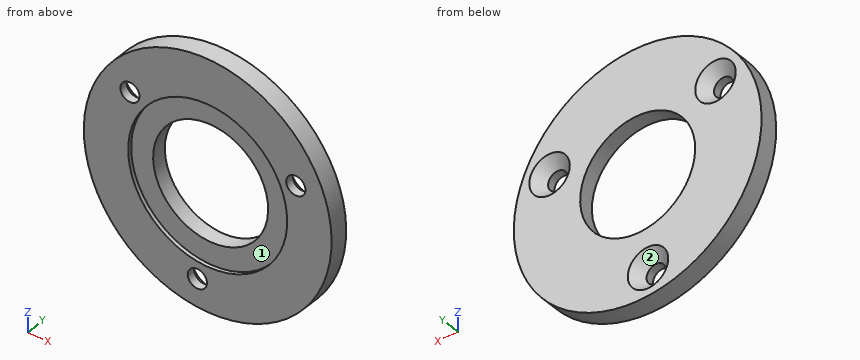
```python
from build123d import *

# Parameters (mm, degrees)
CSK_FOR_M3_SFHCS1_AT_2_COUNT = 2
CSK_FOR_M3_SFHCS1_AT_2_PITCH = 16.002
CSK_FOR_M3_SFHCS1_AT_3_COUNT = 2
CSK_FOR_M3_SFHCS1_AT_3_PITCH = 16.002
CSK_FOR_M3_SFHCS1_AT_4_COUNT = 2
CSK_FOR_M3_SFHCS1_AT_4_PITCH = 16.002


with BuildPart() as part:
    # Sketch1 → Revolve1 (revolve)
    with BuildSketch(Plane.XY, mode=Mode.PRIVATE) as revolve1_sk:
        Polygon((-9.5504, 0), (-20.574, 0), (-20.574, -3.1496), (-13.208, -3.1496), (-13.208, -2.5146), (-9.5504, -2.5146), align=None)
    revolve(revolve1_sk.sketch.rotate(Axis((0, 0, 0), (0, 1, 0)), 270), axis=Axis((0, 0, 0), (0, 1, 0)))

    # Sketch2 → CSK for M3 SFHCS1 (revolve, cut)
    with BuildSketch(Plane(origin=(0, 0, 0), x_dir=(0, 0, 1), z_dir=(1, 0, 0))):
        Polygon((0, 0), (0, 3.1496), (1.6, 3.1496), (1.6, 1.76), (3.36, 0), align=None)
    csk_for_m3_sfhcs1 = revolve(axis=Axis((0, 6.35, 0), (0, -1, 0)), mode=Mode.SUBTRACT)

    # CSK for M3 SFHCS1 at 2: CSK for M3 SFHCS1 ×2
    with Locations(*[Vector(-0.10721238743656843, 0, -0.9942361409545275) * (i * CSK_FOR_M3_SFHCS1_AT_2_PITCH) for i in range(1, CSK_FOR_M3_SFHCS1_AT_2_COUNT)]):
        add(csk_for_m3_sfhcs1, mode=Mode.SUBTRACT)

    # CSK for M3 SFHCS1 at 3: CSK for M3 SFHCS1 ×2
    with Locations(*[Vector(0.9146399491455367, 0, 0.4042694193567579) * (i * CSK_FOR_M3_SFHCS1_AT_3_PITCH) for i in range(1, CSK_FOR_M3_SFHCS1_AT_3_COUNT)]):
        add(csk_for_m3_sfhcs1, mode=Mode.SUBTRACT)

    # CSK for M3 SFHCS1 at 4: CSK for M3 SFHCS1 ×2
    with Locations(*[Vector(-0.8074275617089052, 0, 0.5899667215977628) * (i * CSK_FOR_M3_SFHCS1_AT_4_PITCH) for i in range(1, CSK_FOR_M3_SFHCS1_AT_4_COUNT)]):
        add(csk_for_m3_sfhcs1, mode=Mode.SUBTRACT)


solid = part.part
```
Build history of the part. All positions in model axes, mm. Face numbers are marked on the shaded views. A direction names the side the tool comes from. Round coordinates to 2 decimals unless told otherwise and drop trailing zeros. Order: outer loops, then holes, each group sorted by start corner. A loop starts at its lowest first (then second) coordinate and runs counter-clockwise, first axis right, second up. Notation, with made-up numbers: (28, 0.5) -> (74, 0.5) arc R21 cw to (74, 17.5) -> close; hole circle Ø10 at (-28, 39). An arc over 180 degrees is marked (long way). Answer in a Markdown table with one row per item.
1) Band-saw the part on D-D on z = -11.5. Give the cut face in (x, y), and give its area (3 significant figures).
Values:
| item | result |
|---|---|
| outline | (-17.06, -3.15) -> (-6.5, -3.15) -> (-6.5, -2.51) -> (6.5, -2.51) -> (6.5, -3.15) -> (17.06, -3.15) -> (17.06, 0) -> (-17.06, 0) -> close |
| area | 99.2 mm2 |
2) Band-saw the part on C-C on y = -0.7. Give the cut face in (x, z).
Values:
| item | result |
|---|---|
| outline | circle Ø41.15 at (0, 0); hole circle Ø5.32 at (-12.92, 9.44); hole circle Ø19.1 at (0, 0); hole circle Ø5.32 at (-1.72, -15.91); hole circle Ø5.32 at (14.64, 6.47) |
3) Band-saw the part on B-B on x = 8.5. Give the cut face in (y, z).
Values:
| item | result |
|---|---|
| outline | (-3.15, -18.74) -> (0, -18.74) -> (0, -4.35) -> (-2.51, -4.35) -> (-2.51, -10.11) -> (-3.15, -10.11) -> close; (-3.15, 10.11) -> (-2.51, 10.11) -> (-2.51, 4.35) -> (0, 4.35) -> (0, 18.74) -> (-3.15, 18.74) -> close |
4) Pin check, flat tips, straight feed: P1, Ø2.5, axis at x = -1.72, z = -15.91, coming from the -Y side; P2, Ø1.5, axis at y = -1, z = -6, coming from the +X side. Stop position of each tip, or through.
Values:
| item | result |
|---|---|
| P1 | through |
| P2 | x = 19.89 |
5) Which spindle directions (+Z, -Z, +X, -X, +Y, -Y) get a long thin tool onto all of the face, cutting with end or side? Do the marked faces 1 and 2. Say none if no direction does.
Values:
| item | result |
|---|---|
| face 1 | -Y |
| face 2 | +Y |
6) Band-saw the part on A-A on z = 0. Give the cut face in (x, y).
Values:
| item | result |
|---|---|
| outline | (-20.57, -3.15) -> (-13.21, -3.15) -> (-13.21, -2.51) -> (-9.55, -2.51) -> (-9.55, 0) -> (-20.57, 0) -> close; (9.55, -2.51) -> (13.21, -2.51) -> (13.21, -3.15) -> (20.57, -3.15) -> (20.57, 0) -> (9.55, 0) -> close |
7) Wall check: L1, parallel to X at y = -1.45, z = 7; L2, parallel to X at y = -3, z = 0; L3, parallel to Z at x = -1.5, y = -2.85. Give the ranges that are in metal, low to high.
Values:
| item | result |
|---|---|
| L1 | -19.35 to -6.5, 6.5 to 12.8, 16.47 to 19.35 |
| L2 | -20.57 to -13.21, 13.21 to 20.57 |
| L3 | -20.52 to -17.5, -14.32 to -13.12, 13.12 to 20.52 |
